from build123d import *

# Parameters (mm, degrees)
SKETCH024_W             = 5
SKETCH024_H             = 17.4
EXTRUDE021_DEPTH        = 1.5
EXTRUDE021_DEPTH_BACK   = 60
BODY009_PLACEMENT_ANGLE = 30
EXTRUDE020_DEPTH        = 2


with BuildPart() as body009:
    # Sketch024 → Extrude021 (new body, two sides)
    with BuildSketch(Plane.XZ.offset(29)) as extrude021_sk:
        with Locations((10.5, 7.5)):
            Rectangle(SKETCH024_W, SKETCH024_H)
    extrude(amount=EXTRUDE021_DEPTH)
    extrude(extrude021_sk.sketch, amount=-EXTRUDE021_DEPTH_BACK)


with BuildPart() as body009_1:
    # Body009 placement: moved
    add(body009.part.moved(Location((3, 16.3, 28.6))).rotate(Axis((3, 16.3, 28.6), (1, 0, 0)), BODY009_PLACEMENT_ANGLE))


with BuildPart() as cut:
    # Sketch023 → Extrude020 (new body)
    with BuildSketch(Plane(origin=(0, 0, 0), x_dir=(0, -1, 0), z_dir=(-1, 0, 0))):
        Polygon((19, 35), (19, 20), (-6.5, 20), (-21, 28.371579), (-21, 35), align=None)
    extrude(amount=-EXTRUDE020_DEPTH)


with BuildPart() as cut_1:
    # Extrude020 placement: moved
    add(cut.part.moved(Location((10, 0, 0))))

    # Cut: cut Body009
    add(body009_1.part, mode=Mode.SUBTRACT)


solid = cut_1.part
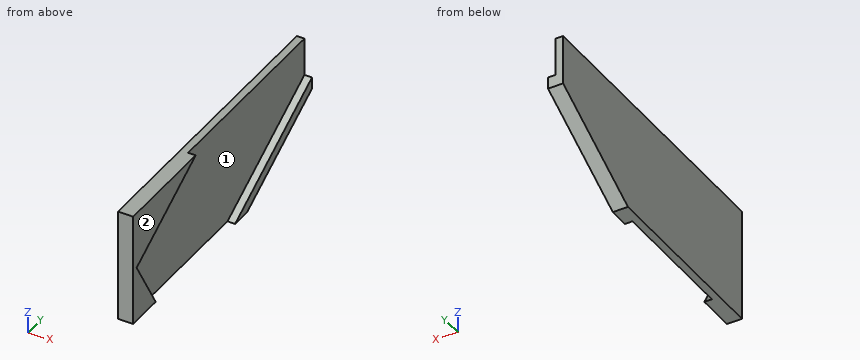
Input: part model. Units: mm. Frame: model coordinates. Face numbers are marked on the shaded views. Give positions to 0.01 mm unless a question says otherwise; leave off trailing zeros. Write each loop counter-clockwise with the first axis right and the second up, starting at its lowest first coordinate (ties: lowest second). Pieces come first, ordered by that corner, then holes.
Q1. Section D-D, the plane z = 24.25. Output: boundary loops of the cut face in (x, y), plus the area to 4 significant figures.
Q2. Section C-C, the plane y = 12.5. Output: boundary loops of the cut face in (x, z).
Q3. Section A-A, the plane x = 11.6. Output: boundary loops of the cut face in (y, z), plus the area to 3 significant figures.
Q4. Section B-B, the plane z = 28. Output: boundary loops of the cut face in (x, y).
Q5. Pull-direction query (Y, two-part tool) for the marked faces 1 and 2; classes: pulls with the +Y half, pulls with the -Y half, needs draft (parallel to the pull), parting line crosses it, or undercut.
Q6. Material intervals for probe 1 along X at (y, z) = (6.5, 32); probe 2 along Y at (x, z) = (11.7, 24.5); probe 3 along Y at (x, z) = (11.2, 25.75), sorted ascending.
Filled in:
1. outline: (10, -19) - (12, -19) - (12, -16.41) - (11, -16.41) - (11, 11.17) - (12, 11.17) - (12, 13.86) - (10, 13.86) - close
1. area: 38.15 mm2
2. outline: (10, 23.46) - (12, 23.46) - (12, 25.02) - (11, 25.02) - (11, 35) - (10, 35) - close
3. outline: (-19, 20) - (-13.95, 20) - (-18.21, 27.38) - (-5.01, 35) - (-19, 35) - close; (3.8, 20) - (6.5, 20) - (21, 28.37) - (21, 29.93) - close
3. area: 102 mm2
4. outline: (10, -19) - (12, -19) - (12, -17.14) - (11, -17.14) - (11, 17.66) - (12, 17.66) - (12, 20.36) - (10, 20.36) - close
5. face 1: undercut
5. face 2: needs draft
6. probe 1: x = 10 to 11
6. probe 2: y = -19 to -16.55, 11.6 to 14.29
6. probe 3: y = -19 to -17.27, 13.76 to 16.46
